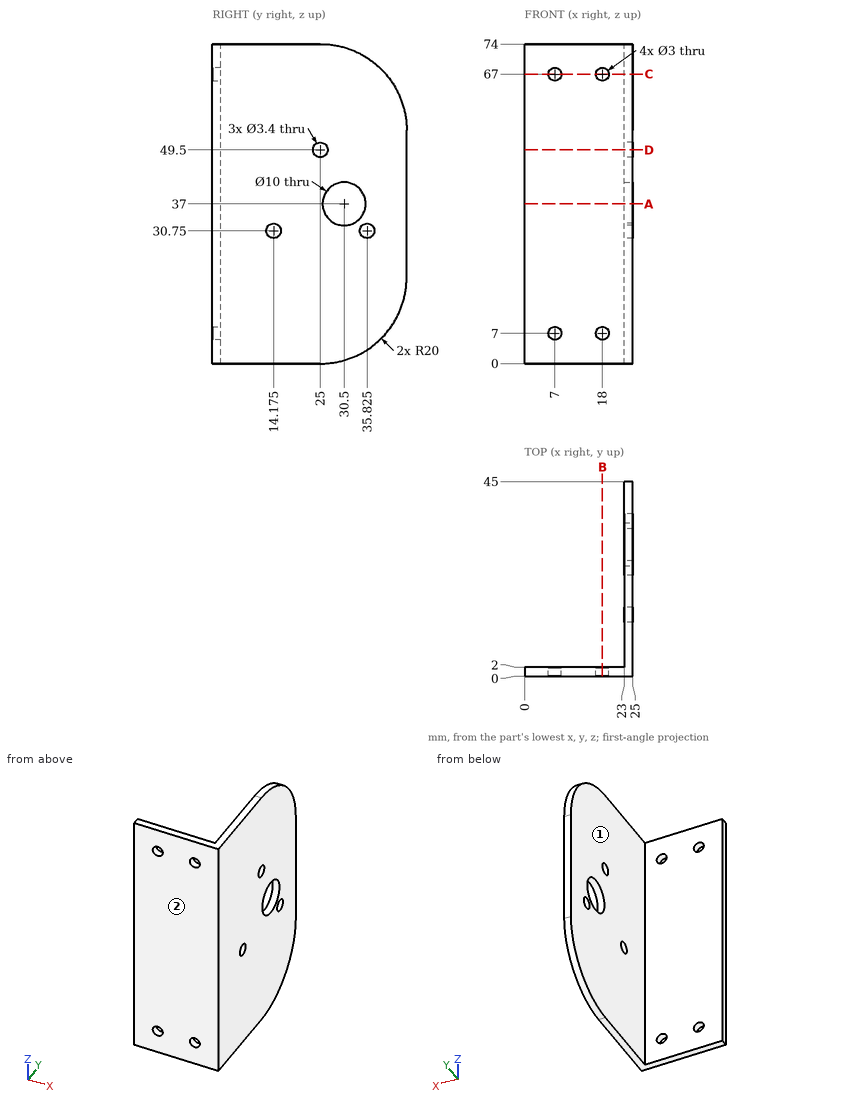
Job drawing, mm, ordinate dimensions from the low corner. One solid piece. A direction names the side the tool comes from. Coordinates: 2 decimals unless noted, no trailing zeros. Write each loop counter-clockwise with the first axis right and the second up, starting at its lowest first coordinate (ties: lowest second). Pieces come first, ordered by that corner, then holes.
Item 1: Slice it at A-A (z = 37). Write the cut outline in (x, y), and give its area (3 significant figures).
Item 2: Which spindle directions (+Z, -Z, +X, -X, +Y, -Y) get a long thin tool onto all of the face, cutting with end or side? Do the marked faces 1 and 2. Say none if no direction does.
Item 3: Slice it at C-C (z = 67). Write the cut outline in (x, y).
Item 4: Slice it at B-B (x = 18). Write the cut outline in (y, z).
Item 5: Probe line 1 (X direction, y = 1.2, z = 7); line 2 (Y direction, x = 23.6, z = 30.75) (1 decimal); line 3 (Y direction, x = 23.95, z = 37). List the from-to ranges inside material, lowest first.
Item 6: Slice it at D-D (z = 49.5). Write the cut outline in (x, y).
Item 7: Pin check, flat tips, straight feed: pin 1 (4 mm diameter, centred on y = 35.83, z = 30.75, fed in from -X); pin 2 (4 mm diameter, centred on x = 20.5, y = 26, fed in from +Z); pin 3 (4 mm diameter, centred on y = 25, z = 49.5, fed in from +X); pin 4 (3.5 mm diameter, centred on x = 18, z = 7, fed in from +Y). Stop position of each tip, or through.
Results found:
1. outline: (0, 0) - (25, 0) - (25, 25.5) - (23, 25.5) - (23, 2) - (0, 2) - close; (23, 35.5) - (25, 35.5) - (25, 45) - (23, 45) - close
1. area: 116 mm2
2. face 1: +Z, -Z, -X, +Y
2. face 2: +Z, -Z, +X, -X, -Y
3. outline: (0, 0) - (5.5, 0) - (5.5, 2) - (0, 2) - close; (8.5, 0) - (16.5, 0) - (16.5, 2) - (8.5, 2) - close; (19.5, 0) - (25, 0) - (25, 40.2) - (23, 40.2) - (23, 2) - (19.5, 2) - close
4. outline: (0, 0) - (2, 0) - (2, 5.5) - (0, 5.5) - close; (0, 8.5) - (2, 8.5) - (2, 65.5) - (0, 65.5) - close; (0, 68.5) - (2, 68.5) - (2, 74) - (0, 74) - close
5. line 1: x = 0 to 5.5, 8.5 to 16.5, 19.5 to 25
5. line 2: y = 0 to 12.5, 15.9 to 34.1, 37.5 to 45
5. line 3: y = 0 to 25.5, 35.5 to 45
6. outline: (0, 0) - (25, 0) - (25, 23.3) - (23, 23.3) - (23, 2) - (0, 2) - close; (23, 26.7) - (25, 26.7) - (25, 45) - (23, 45) - close
7. pin 1: stops at x = 23
7. pin 2: passes through
7. pin 3: stops at x = 25
7. pin 4: stops at y = 2
